Geometry: final body of the model. Coordinates: model frame, mm. A direction names the side the tool comes from. Round coordinates to 2 decimals unless told otherwise and drop trailing zeros. Write each loop counter-clockwise with the first axis right and the second up, starting at its lowest first coordinate (ties: lowest second). Pieces come first, ordered by that corner, then holes. Notation, with made-up numbers: (82.5, 31.25) -> (86.5, 31.25) arc R22 cw to (86.5, 52.25) -> close; hole circle Ø4 at (37.25, -23). An arc over 180 degrees is marked (long way). Use one line per item in the form item = value. Start each with the question number.
1. Line query: L1, parallel to Y at x = 0, z = -2.9; L2, parallel to Z at x = 5.75, y = 3; L3, parallel to Y at x = 3.75, z = 5. Output: solid intervals per line, ascending.
2. Cut plane D-D, the plane z = 2. Return the cut outline in (x, y), plus the area to 3 significant figures.
3. Draft query along Z for faces 4 (the face through (4.98, 2.52, 8.01)), 5 (the face through (10.71, 0, 8)), 6 (the face through (5, 0, 13.8)), 7 (the face through (10, 0, -3.6)). Return one class per face: pulls with the +Z half, pulls with the -Z half, needs draft (parallel to the pull), parting line crosses it, or undercut.
4. Cut plane C-C, the plane x = 1.75. Return the cut outline in (y, z), plus the area to 3 significant figures.
5. Pin query (flat end, axial travel): pin 1 Ø0.9 at (y, z) = (0, -1.5) entering from -X; pin 2 Ø0.6 at (y, z) = (0, 10.5) entering from +X; pin 3 Ø0.6 at (x, z) = (10.5, -2.5) entering from -Y; pin 4 Ø5 at (y, z) = (3.5, 9.5) entering from +X. Return the tip coordinate at first contact, or that it passes through.
6. Reachability of faces 1 (the face through (9.61, 0, -2)), 2 (the face through (4.975, 4.566, 7.335)), 3 (the face through (5.18, 1.55, 9.69)) from +Z, -Z, +X, -X, +Y, -Y: full face, straight path, thin tool, end or side. Return the list, or none.
7. Cut plane A-A, the plane z = 5.25. Return the cut outline in (x, y).
```python
from build123d import *

# Parameters (mm, degrees)
SKETCH_2_W           = 15
SKETCH_2_H           = 10.4
EXTRUDE_1_DEPTH      = 3.2
EXTRUDE_2_DEPTH      = 13.8
EXTRUDE_2_DEPTH_BACK = 3.6
SKETCH_3_W           = 1.1
SKETCH_3_H           = 1.1
SKETCH_5_W           = 15
SKETCH_5_H           = 1.2
SKETCH_6_R           = 0.325501749
CUT_EXTRUDE_1_DEPTH  = 2


with BuildPart() as part:
    # Эскиз2 → Вытянуть1 (new body)
    with BuildSketch(Plane.XY):
        with Locations((5.08, -0.4)):
            Rectangle(SKETCH_2_W, SKETCH_2_H)
    extrude(amount=EXTRUDE_1_DEPTH)

    # Эскиз3 → Вытянуть2 (add, two sides: drawn at the far end of the back side and taken through both)
    with BuildSketch(Plane.XY.offset(-EXTRUDE_2_DEPTH_BACK)):
        Rectangle(SKETCH_3_W, SKETCH_3_H)
        with Locations((5.08, 0)):
            Rectangle(SKETCH_3_W, SKETCH_3_H)
        with Locations((10.16, 0)):
            Rectangle(SKETCH_3_W, SKETCH_3_H)
    extrude(amount=EXTRUDE_2_DEPTH + EXTRUDE_2_DEPTH_BACK)

    # По траектории1: sweep along a path in Эскиз4
    with BuildLine(Plane.ZY.offset(2.42)) as sweep_1_path:
        Line((3.2, 4.2), (6.152565934, 4.2))
        ThreePointArc((6.152565934, 4.2), (7.118635036, 4.005799317), (7.934615114, 3.453368392))
        Line((7.934615114, 3.453368392), (8.923160693, 2.448652643))
        ThreePointArc((8.923160693, 2.448652643), (9.678881269, 2.150920668), (10.406297634, 2.512339193))
        Line((10.406297634, 2.512339193), (12.3, 4.8))
    # Эскиз5 → По траектории1 (sweep)
    with BuildSketch(Plane.XY.offset(3.2)):
        with Locations((5.08, 4.2)):
            Rectangle(SKETCH_5_W, SKETCH_5_H)
    sweep(path=sweep_1_path.line)

    # Эскиз6 → Вырез-Вытянуть1 (cut)
    with BuildSketch(Plane(origin=(0, 0, -3.6), x_dir=(-1, 0, 0), z_dir=(0, 0, -1))):
        Circle(SKETCH_6_R)
    extrude(amount=-CUT_EXTRUDE_1_DEPTH, mode=Mode.SUBTRACT)


solid = part.part
```
Outcome:
q1.L1 = -0.55 to -0.33, 0.33 to 0.55
q1.L2 = 0 to 3.2, 7.54 to 9.22, 10.03 to 11.59
q1.L3 = 3.6 to 4.8
q2.outline = (-2.42, -5.6) -> (12.58, -5.6) -> (12.58, 4.8) -> (-2.42, 4.8) -> close
q2.area = 156 mm^2
q3.face_4 = undercut
q3.face_5 = needs draft
q3.face_6 = pulls with the +Z half
q3.face_7 = pulls with the -Z half
q4.outline = (-5.6, 0) -> (4.8, 0) -> (4.8, 6.15) arc R3.1 ccw to (3.87, 8.36) -> (2.87, 9.35) arc R0.4 cw to (2.89, 9.94) -> (5.18, 11.84) -> (4.42, 12.76) -> (2.13, 10.87) arc R1.6 ccw to (2.03, 8.5) -> (3.03, 7.51) arc R1.9 cw to (3.6, 6.15) -> (3.6, 3.2) -> (-5.6, 3.2) -> close
q4.area = 46.5 mm^2
q5.pin_1 = -0.55
q5.pin_2 = 10.71
q5.pin_3 = -0.55
q5.pin_4 = 12.58
q6.face_1 = -Z, +Y, -Y
q6.face_2 = +X, -X, +Y
q6.face_3 = +X, -X
q7.outline = (-2.42, 3.6) -> (12.58, 3.6) -> (12.58, 4.8) -> (-2.42, 4.8) -> close; (-0.55, -0.55) -> (0.55, -0.55) -> (0.55, 0.55) -> (-0.55, 0.55) -> close; (4.53, -0.55) -> (5.63, -0.55) -> (5.63, 0.55) -> (4.53, 0.55) -> close; (9.61, -0.55) -> (10.71, -0.55) -> (10.71, 0.55) -> (9.61, 0.55) -> close
